from build123d import *

# Parameters (mm, degrees)
CYLINDER167_R               = 0.9
CYLINDER167_DEPTH           = 6
CYLINDER168_R               = 0.9
CYLINDER168_DEPTH           = 6
CYLINDER166_R               = 1.1
CYLINDER166_DEPTH           = 10
CYLINDER166_PLACEMENT_ANGLE = 75
CYLINDER165_R               = 3.1
CYLINDER165_DEPTH           = 4
CYLINDER163_R               = 1.6
CYLINDER163_DEPTH           = 10
CYLINDER164_R               = 3.1
CYLINDER164_DEPTH           = 4
CYLINDER162_R               = 1.6
CYLINDER162_DEPTH           = 10
CYLINDER160_R               = 5
CYLINDER160_DEPTH           = 180
BOX077_W                    = 20
BOX077_H                    = 10
BOX077_DEPTH                = 10
BOX076_W                    = 21
BOX076_H                    = 10
BOX076_DEPTH                = 10
FILLET039_R                 = 3
BOX074_W                    = 21
BOX074_H                    = 10
BOX074_DEPTH                = 10
BOX073_W                    = 10
BOX073_H                    = 10
BOX073_DEPTH                = 25
BOX073_PLACEMENT_ANGLE      = 3
BOX075_W                    = 10
BOX075_H                    = 10
BOX075_DEPTH                = 54
BOX075_PLACEMENT_ANGLE      = 15
FILLET040_R                 = 2
FILLET041_R                 = 5


with BuildPart() as cylinder167:
    # Cylinder167 → Cylinder167 (new body)
    with BuildSketch(Plane(origin=(605, 11, -7), x_dir=(1, 0, 0), z_dir=(0, -1, 0))):
        Circle(CYLINDER167_R)
    extrude(amount=CYLINDER167_DEPTH)


with BuildPart() as fusion145:
    # Cylinder168 → Cylinder168 (new body)
    with BuildSketch(Plane(origin=(605, 11, 0), x_dir=(1, 0, 0), z_dir=(0, -1, 0))):
        Circle(CYLINDER168_R)
    extrude(amount=CYLINDER168_DEPTH)

    # Fusion145: union Cylinder167
    add(cylinder167.part)


with BuildPart() as fusion145_1:
    # Fusion145 placement: moved
    add(fusion145.part.moved(Location((0, -4, 0))))


with BuildPart() as cylinder166:
    # Cylinder166 → Cylinder166 (new body)
    with BuildSketch(Plane.XY):
        Circle(CYLINDER166_R)
    extrude(amount=CYLINDER166_DEPTH)


with BuildPart() as cylinder166_1:
    # Cylinder166 placement: moved
    add(cylinder166.part.moved(Location((604.475462, 6, -27.270932))).rotate(Axis((604.475462, 6, -27.270932), (0, 1, 0)), CYLINDER166_PLACEMENT_ANGLE))


with BuildPart() as cylinder165:
    # Cylinder165 → Cylinder165 (new body)
    with BuildSketch(Plane(origin=(606, 7, 6), x_dir=(0, 0, -1), z_dir=(1, 0, 0))):
        Circle(CYLINDER165_R)
    extrude(amount=CYLINDER165_DEPTH)


with BuildPart() as cylinder163:
    # Cylinder163 → Cylinder163 (new body)
    with BuildSketch(Plane(origin=(599, 7, 6), x_dir=(0, 0, -1), z_dir=(1, 0, 0))):
        Circle(CYLINDER163_R)
    extrude(amount=CYLINDER163_DEPTH)


with BuildPart() as cylinder164:
    # Cylinder164 → Cylinder164 (new body)
    with BuildSketch(Plane(origin=(604, 7, 14), x_dir=(0, 0, -1), z_dir=(1, 0, 0))):
        Circle(CYLINDER164_R)
    extrude(amount=CYLINDER164_DEPTH)


with BuildPart() as fusion144:
    # Cylinder162 → Cylinder162 (new body)
    with BuildSketch(Plane(origin=(599, 7, 14), x_dir=(0, 0, -1), z_dir=(1, 0, 0))):
        Circle(CYLINDER162_R)
    extrude(amount=CYLINDER162_DEPTH)

    # Fusion144: union Cylinder165, Cylinder163, Cylinder164
    add(cylinder165.part)
    add(cylinder163.part)
    add(cylinder164.part)


with BuildPart() as cylinder160:
    # Cylinder160 → Cylinder160 (new body)
    with BuildSketch(Plane(origin=(615, 121, -24), x_dir=(1, 0, 0), z_dir=(0, -1, 0))):
        Circle(CYLINDER160_R)
    extrude(amount=CYLINDER160_DEPTH)


with BuildPart() as box077:
    # Box077 → Box077 (new body)
    with BuildSketch(Plane(origin=(603, 1, -41), x_dir=(1, 0, 0), z_dir=(0, 0, 1))):
        with Locations((10, 5)):
            Rectangle(BOX077_W, BOX077_H)
    extrude(amount=BOX077_DEPTH)


with BuildPart() as fillet039:
    # Box076 → Box076 (new body)
    with BuildSketch(Plane(origin=(591, 1, 8.5), x_dir=(1, 0, 0), z_dir=(0, 0, 1))):
        with Locations((10.5, 5)):
            Rectangle(BOX076_W, BOX076_H)
    extrude(amount=BOX076_DEPTH)

    # Fillet039
    fillet039_edges = [fillet039.edges().sort_by_distance(p)[0] for p in [
        (601.5, 1, 18.5),
    ]]
    fillet(fillet039_edges, radius=FILLET039_R)


with BuildPart() as cut088:
    # Box074 → Box074 (new body)
    with BuildSketch(Plane(origin=(591, 1, 15.5), x_dir=(1, 0, 0), z_dir=(0, 0, 1))):
        with Locations((10.5, 5)):
            Rectangle(BOX074_W, BOX074_H)
    extrude(amount=BOX074_DEPTH)

    # Cut088: cut Fillet039
    add(fillet039.part, mode=Mode.SUBTRACT)


with BuildPart() as fusion143:
    # Box073 → Box073 (new body)
    with BuildSketch(Plane.XY):
        with Locations((5, 5)):
            Rectangle(BOX073_W, BOX073_H)
    extrude(amount=BOX073_DEPTH)


with BuildPart() as fusion143_1:
    # Box073 placement: moved
    add(fusion143.part.moved(Location((590, 1, -2))).rotate(Axis((590, 1, -2), (0, -1, 0)), BOX073_PLACEMENT_ANGLE))

    # Fusion143: union Cut088
    add(cut088.part)


with BuildPart() as left_bumper_holder:
    # Box075 → Box075 (new body)
    with BuildSketch(Plane.XY):
        with Locations((5, 5)):
            Rectangle(BOX075_W, BOX075_H)
    extrude(amount=BOX075_DEPTH)


with BuildPart() as left_bumper_holder_1:
    # Box075 placement: moved
    add(left_bumper_holder.part.moved(Location((609, 1, -33))).rotate(Axis((609, 1, -33), (0, -1, 0)), BOX075_PLACEMENT_ANGLE))

    # Cut089: cut Fusion143
    add(fusion143_1.part, mode=Mode.SUBTRACT)

    # Cut090: cut Box077
    add(box077.part, mode=Mode.SUBTRACT)

    # Fillet040
    fillet040_edges = [left_bumper_holder_1.edges().sort_by_distance(p)[0] for p in [
        (618.659258, 6, -30.41181),
    ]]
    fillet(fillet040_edges, radius=FILLET040_R)

    # Fillet041
    fillet041_edges = [left_bumper_holder_1.edges().sort_by_distance(p)[0] for p in [
        (608.464102, 6, -31),
    ]]
    fillet(fillet041_edges, radius=FILLET041_R)

    # Cut091: cut Cylinder160
    add(cylinder160.part, mode=Mode.SUBTRACT)

    # Cut092: cut Fusion144
    add(fusion144.part, mode=Mode.SUBTRACT)

    # Cut093: cut Cylinder166
    add(cylinder166_1.part, mode=Mode.SUBTRACT)

    # Cut094: cut Fusion145
    add(fusion145_1.part, mode=Mode.SUBTRACT)


with BuildPart() as left_bumper_holder_2:
    # Cut094 placement: moved
    add(left_bumper_holder_1.part.moved(Location((0, -10, 0))))


solid = left_bumper_holder_2.part
Check sheet for the modelled part. Datum: model origin and axes. Units: mm. A direction names the side the tool comes from. Give positions to 0.01 mm unless a question says otherwise; leave off trailing zeros. Write each loop counter-clockwise with the first axis right and the second up, starting at its lowest first coordinate (ties: lowest second). Pieces come first, ordered by that corner, then holes. Notation, with made-up numbers: M 42.25,10.25 L 86.25,10.25 A21 ccw 86.25,37.25 Z; hole C 67,-14 d2. An arc over 180 degrees is marked long. Use one line per item in the form item = value.
(1) Depth check by flat-ended pin: P1, Ø3, axis at y = -5.5, z = -6.5, coming from the -X side; P2, Ø5, axis at y = -3, z = 14, coming from the -X side; P3, Ø3, axis at y = -3, z = 13, coming from the +X side. Enter the tip coordinate at first touch or a pass-through.
Answer block:
P1 = 601.5
P2 = 599.04
P3 = 604
(2) Section check C-C on y = -7.75. Record the boundary of the cut face in (x, z), plus the area to 3 significant figures.
Answer block:
outline = M 598.97,17.94 L 599.85,1.15 L 607.47,-27.29 A5 ccw 612.3,-31 L 616.46,-31 L 616.73,-30.93 A2 ccw 618.14,-28.48 L 618.01,-27.99 A5 cw long 615.61,-19.04 L 605.7,17.94 Z; hole C 605,-7 d1.8; hole C 605,0 d1.8
area = 409 mm2
(3) Draft check along Z on faces 4 (the cylindrical face through (617.93, -3.93, -30.02)), 5 (the cylindrical face through (609.3, -3.9, -30)), 6 (the cylindrical face through (605.371, -2.069, 11.043)), 7 (the cylindrical face through (601.51, -2.93, 15.6)). Enter one of: pulls with the +Z half, pulls with the -Z half, needs draft (parallel to the pull), parting line crosses it, or undercut.
Answer block:
face_4 = parting line crosses it
face_5 = pulls with the -Z half
face_6 = undercut
face_7 = undercut
(4) Tool access check on faces 1 (the cylindrical face through (609.139, -3.67, -27.107)), 2 (the flat face through (606, -4.3, 4.7)), 3 (the cylindrical face through (604.1, -6, -7)). Record the directions out of +Z, -Z, +X, -X, +Y, -Y that give a thin tool (end or side, any length) a straight path to the whole face; none if there is none.
Answer block:
face_1 = none
face_2 = +X
face_3 = -Y
(5) Section check D-D on x = 600.5. Record the boundary of the cut face in (y, z).
Answer block:
outline = M -9,-1.28 L 1,-1.28 L 1,18.5 L -6,18.5 A3 ccw -9,15.5 Z; hole C -3,6 d3.2; hole C -3,14 d3.2
(6) Material ranges on line 1 along Y through (x, z) = (604.8, 14); line 2 along X through (y, z) = (-7, 16); line 3 along X through (y, z) = (0.5, -11.5), recorded low to high.
Answer block:
line_1 = -9 to -6.1, 0.1 to 1
line_2 = 599.07 to 606.22
line_3 = 603.24 to 613.59
(7) Section check B-B on x = 611.5. Record the boundary of the cut face in (y, z).
Answer block:
outline = M -9,-30.94 L 1,-30.94 L 1,-27.57 L -9,-27.57 Z; M -9,-20.43 L 1,-20.43 L 1,-3.69 L -9,-3.69 Z
(8) Section check A-A on z = 6. Record the boundary of the cut face in (x, y).
Answer block:
outline = M 599.59,-9 L 608.9,-9 L 608.9,-6.1 L 606,-6.1 L 606,-4.6 L 599.59,-4.6 Z; M 599.59,-1.4 L 606,-1.4 L 606,0.1 L 608.9,0.1 L 608.9,1 L 599.59,1 Z
